Check sheet for the modelled part. Datum: model origin and axes. Units: mm. Round coordinates to 2 decimals unless told otherwise and drop trailing zeros. Order: outer loops, then holes, each group sorted by start corner. A loop starts at its lowest first (then second) coordinate and runs counter-clockwise, first axis right, second up.
```python
from build123d import *

# Parameters (mm, degrees)
ESQUISSE1_W             = 120
ESQUISSE1_H             = 120
ESQUISSE1_R             = 1.25
ESQUISSE1_R_2           = 12.7
BOSS_EXTRU_1_DEPTH      = 6.35
CONG_1_R                = 2
ESQUISSE2_R             = 1.65
ENL_V_MAT_EXTRU_1_DEPTH = 7.35


with BuildPart() as part:
    # Esquisse1 → Boss.-Extru.1 (new body)
    with BuildSketch(Plane.XY):
        with Locations((60, 60)):
            Rectangle(ESQUISSE1_W, ESQUISSE1_H)
        with Locations((7.5, 112.5)):
            Circle(ESQUISSE1_R, mode=Mode.SUBTRACT)
        with Locations((112.5, 112.5)):
            Circle(ESQUISSE1_R, mode=Mode.SUBTRACT)
        with Locations((112.5, 7.5)):
            Circle(ESQUISSE1_R, mode=Mode.SUBTRACT)
        with Locations((7.5, 7.5)):
            Circle(ESQUISSE1_R, mode=Mode.SUBTRACT)
        with Locations((60, 60)):
            Circle(ESQUISSE1_R_2, mode=Mode.SUBTRACT)
    extrude(amount=BOSS_EXTRU_1_DEPTH)

    # Congé1
    cong_1_edges = [part.edges().sort_by_distance(p)[0] for p in [
        (0, 120, 3.175),
        (120, 120, 3.175),
        (120, 0, 3.175),
        (0, 0, 3.175),
    ]]
    fillet(cong_1_edges, radius=CONG_1_R)

    # Esquisse2 → Enlèv. mat.-Extru.1 (cut, through all)
    with BuildSketch(Plane.XY.offset(6.35)):
        with Locations((60, 85.4)):
            Circle(ESQUISSE2_R)
        with Locations((38.002954744, 47.3)):
            Circle(ESQUISSE2_R)
        with Locations((81.997045256, 47.3)):
            Circle(ESQUISSE2_R)
    extrude(amount=-ENL_V_MAT_EXTRU_1_DEPTH, mode=Mode.SUBTRACT)


solid = part.part
```
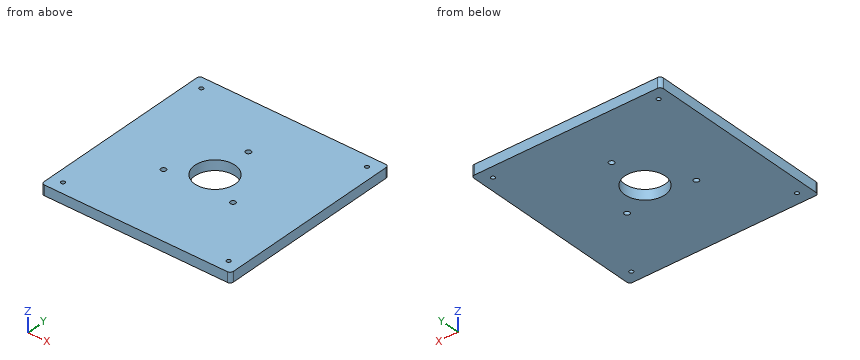
Item 1: Sectioned sample at B-B (x = 60). Record the cut outline in (y, z).
Answer:
outline: (0, 0) - (47.3, 0) - (47.3, 6.35) - (0, 6.35) - close; (72.7, 0) - (83.75, 0) - (83.75, 6.35) - (72.7, 6.35) - close; (87.05, 0) - (120, 0) - (120, 6.35) - (87.05, 6.35) - close
Item 2: Go/stop test with flat-tipped pins: P1, Ø4.5, axis at x = 38, y = 47.3, coming from the -Z side; P2, Ø3, axis at x = 60, y = 85.4, coming from the +Z side (3 decimals). Record where each tip stops, or that it passes through.
Answer:
P1: stops at z = 0
P2: passes through
Item 3: Scan lines: line 1 along Y through (x, z) = (7.5, 5.25); line 2 along X through (y, z) = (85.5, 4). Record each from-to range of solid material in increasing order.
Answer:
line 1: y = 0 to 6.25, 8.75 to 111.25, 113.75 to 120
line 2: x = 0 to 58.35, 61.65 to 120
Item 4: Sectioned sample at A-A (y = 85.4). Record the cut outline in (x, z), and give its area (3 significant figures).
Answer:
outline: (0, 0) - (58.35, 0) - (58.35, 6.35) - (0, 6.35) - close; (61.65, 0) - (120, 0) - (120, 6.35) - (61.65, 6.35) - close
area: 741 mm2
Item 5: Sectioned sample at C-C (z = 3). State how many separate pieces and enclosed holes the cut face has, and give its area (3 significant figures).
Answer:
separate pieces: 1
enclosed holes: 8
area: 13,800 mm2
